Answer from the drawing. Dimensions are ordinates in mm from the lowest x, y and z of the part. Round coordinates to 2 decimals unless told otherwise and drop trailing zeros. Loops run counter-clockwise (first coordinate to the right, second up) from the corner with the lowest first, then second, coordinate; pieces in that order, holes last. Notation, with made-up numbers: M 34.5,29 L 91.5,29 A21 ccw 91.5,49 Z; hole C -29,-21.75 d10. An arc over 180 degrees is marked long. One line per item, written item: value.
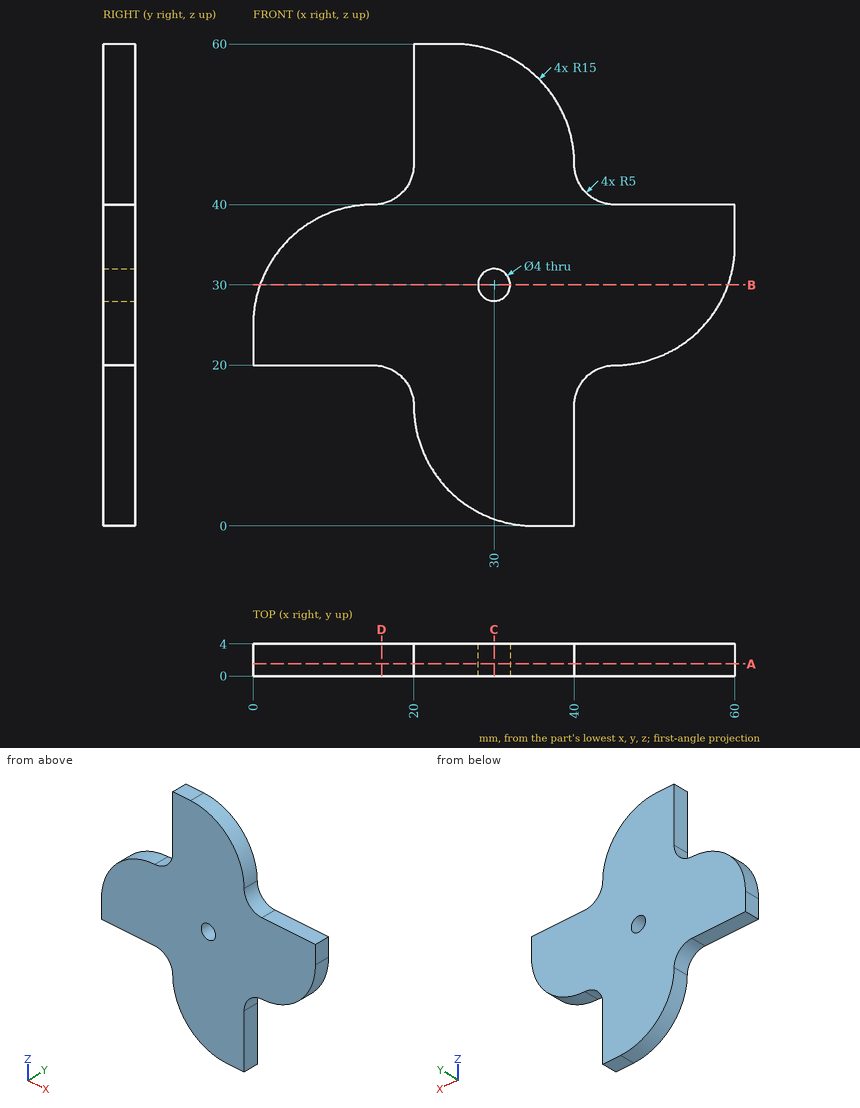
1) Find the intervals of material crossed by probe 1 along Z at (x, y) = (30, 1.4); probe 2 along Z at (x, y) = (28.5, 0.7); probe 3 along X at (y, z) = (0.55, 53), in increasing order. Write a range as from..to.
Check values:
probe 1: 0.86..28, 32..59.14
probe 2: 1.48..28.68, 31.32..59.59
probe 3: 20..37.69
2) Find section D-D (x = 16). Give the vertices of the cut face in (y, z), then the cut area to 3 significant figures.
Check values:
outline: M 0,19.9 L 4,19.9 L 4,40.1 L 0,40.1 Z
area: 80.8 mm2
3) Find section A-A (y = 1.5). Give the vertices of the cut face in (x, z).
Check values:
outline: M 0,20 L 15,20 A5 cw 20,15 A15 ccw 35,0 L 40,0 L 40,15 A5 cw 45,20 A15 ccw 60,35 L 60,40 L 45,40 A5 cw 40,45 A15 ccw 25,60 L 20,60 L 20,45 A5 cw 15,40 A15 ccw 0,25 Z; hole C 30,30 d4
4) This flat-tipped pin is pushed along its axis until it touches: pin 1 (2 mm diameter, centred on y = 2, z = 51.5, fed in from -X). Where does it stop, or does it pass through?
Check values:
pin 1: x = 20
5) Find section C-C (x = 30). Give the vertices of the cut face in (y, z).
Check values:
outline: M 0,0.86 L 4,0.86 L 4,28 L 0,28 Z; M 0,32 L 4,32 L 4,59.14 L 0,59.14 Z
6) Find section B-B (z = 30). Give the vertices of the cut face in (x, y).
Check values:
outline: M 0.86,0 L 28,0 L 28,4 L 0.86,4 Z; M 32,0 L 59.14,0 L 59.14,4 L 32,4 Z
